```python
from build123d import *

# Parameters (mm, degrees)
MAIN_SHAPE_DEPTH = 0.6
FILLET1_R        = 15


with BuildPart() as part:
    # Sketch2 → Main Shape (new body)
    with BuildSketch(Plane.XY):
        with BuildLine():
            Line((-14, -91.764766734), (14, -91.764766734))
            Line((14, -91.764766734), (68.266232563, -84.05670244))
            ThreePointArc((68.266232563, -84.05670244), (74.651075824, -82.937586842), (80.95, -81.407162906))
            Line((80.95, -81.407162906), (80.95, -49.66))
            Line((80.95, -49.66), (82.95, -49.66))
            Line((82.95, -49.66), (82.95, -52.66))
            Line((82.95, -52.66), (84.95, -52.66))
            Line((84.95, -52.66), (88.95, -49.66))
            Line((88.95, -49.66), (88.95, -47.66))
            Line((88.95, -47.66), (80.95, -44.66))
            Line((80.95, -44.66), (80.95, -42.66))
            Line((80.95, -42.66), (88.95, -39.66))
            Line((88.95, -39.66), (88.95, -37.66))
            Line((88.95, -37.66), (84.95, -34.66))
            Line((84.95, -34.66), (82.95, -34.66))
            Line((82.95, -34.66), (82.95, -37.66))
            Line((82.95, -37.66), (80.95, -37.66))
            Line((80.95, -37.66), (80.95, -18.389599053))
            Line((80.95, -18.389599053), (50.74391922, -13.264766734))
            ThreePointArc((50.74391922, -13.264766734), (40.804108255, -9.246591688), (33.461443341, -1.434367632))
            ThreePointArc((33.461443341, -1.434367632), (26.448172688, 5.805997675), (16.941855461, 9.15842781))
            Line((16.941855461, 9.15842781), (7, 10.235233266))
            Line((7, 10.235233266), (0, 0))
            Line((0, 0), (-7, 10.235233266))
            Line((-7, 10.235233266), (-16.941855461, 9.15842781))
            ThreePointArc((-16.941855461, 9.15842781), (-26.448172688, 5.805997675), (-33.461443341, -1.434367632))
            ThreePointArc((-33.461443341, -1.434367632), (-40.804108255, -9.246591688), (-50.74391922, -13.264766734))
            Line((-50.74391922, -13.264766734), (-80.95, -18.389599053))
            Line((-80.95, -18.389599053), (-80.95, -37.66))
            Line((-80.95, -37.66), (-82.95, -37.66))
            Line((-82.95, -37.66), (-82.95, -34.66))
            Line((-82.95, -34.66), (-84.95, -34.66))
            Line((-84.95, -34.66), (-88.95, -37.66))
            Line((-88.95, -37.66), (-88.95, -39.66))
            Line((-88.95, -39.66), (-80.95, -42.66))
            Line((-80.95, -42.66), (-80.95, -44.66))
            Line((-80.95, -44.66), (-88.95, -47.66))
            Line((-88.95, -47.66), (-88.95, -49.66))
            Line((-88.95, -49.66), (-84.95, -52.66))
            Line((-84.95, -52.66), (-82.95, -52.66))
            Line((-82.95, -52.66), (-82.95, -49.66))
            Line((-82.95, -49.66), (-80.95, -49.66))
            Line((-80.95, -49.66), (-80.95, -81.407162906))
            ThreePointArc((-80.95, -81.407162906), (-74.651075824, -82.937586842), (-68.266232563, -84.05670244))
            Line((-68.266232563, -84.05670244), (-14, -91.764766734))
        make_face()
    extrude(amount=MAIN_SHAPE_DEPTH)

    # Fillet1
    fillet1_edges = [part.edges().sort_by_distance(p)[0] for p in [
        (80.95, -18.389599053, 0.3),
        (-80.95, -18.389599053, 0.3),
    ]]
    fillet(fillet1_edges, radius=FILLET1_R)


solid = part.part
```
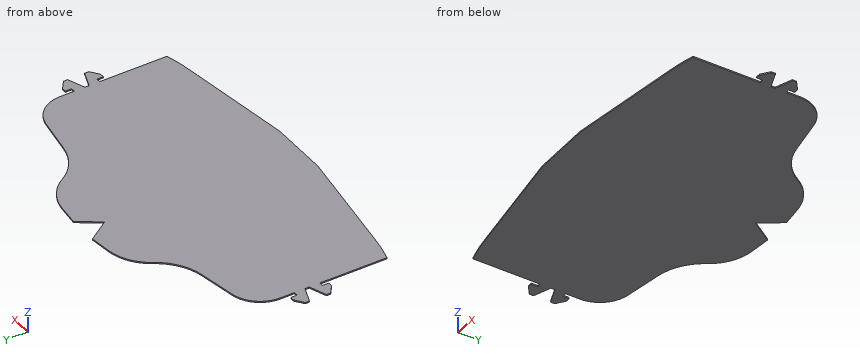
Design review of the part built by this model. Coordinates are the model's own, in mm. Give positions to 0.01 mm unless a question says otherwise; leave off trailing zeros. Order: outer loops, then holes, each group sorted by start corner. A loop starts at its lowest first (then second) coordinate and runs counter-clockwise, first axis right, second up. Notation, with made-up numbers: (28.25, 60) -> (68.25, 60) arc R20 cw to (68.25, 75) -> close; hole circle Ø10 at (88.5, 2.25). An arc over 180 degrees is marked (long way). Write each question's results on one line, items separated by ' | '. Start each with the question number.
Q1. Add section C-C on y = -24.5. Give the boundary of the cut face in (x, z), and give its area (3 significant figures).
Q2. For pin 1 (6 mm diameter, centred on x = 67, y = -70.5, fed in from -Z), flat-tipped, find the tip position at first contact; note if it passes through.
Q3. Add section A-A on y = 2.5. Give the boundary of the cut face in (x, z).
Q4. Add section B-B on x = 36. Give the boundary of the cut face in (y, z).
Q5. Wall thickness on L1, parallel to X at y = 1.5, z = 0.5; L2, parallel to X at y = -63, z = 0.5; L3, parallel to X at y = 2, z = 0.35: over which ranges is each line inside the solid? List them lowest first. Write a range as from..to.
Found:
1) outline: (-79.44, 0) -> (79.44, 0) -> (79.44, 0.6) -> (-79.44, 0.6) -> close | area: 95.3 mm2
2) pin 1: stops at z = 0
3) outline: (-30.46, 0) -> (-1.71, 0) -> (-1.71, 0.6) -> (-30.46, 0.6) -> close; (1.71, 0) -> (30.46, 0) -> (30.46, 0.6) -> (1.71, 0.6) -> close
4) outline: (-88.64, 0) -> (-4.95, 0) -> (-4.95, 0.6) -> (-88.64, 0.6) -> close
5) L1: x = -31.36..-1.03, 1.03..31.36 | L2: x = -80.95..80.95 | L3: x = -30.93..-1.37, 1.37..30.93
